Verification items for this drawing (mm, ordinates from the low corner). Round coordinates to 2 decimals unless told otherwise and drop trailing zeros. Order: outer loops, then holes, each group sorted by start corner. A loop starts at its lowest first (then second) coordinate and runs counter-clockwise, first axis right, second up. Notation, with made-up numbers: (61, 21) -> (106, 21) arc R17 cw to (106, 29) -> close; hole circle Ø2 at (35.5, 4). An arc over 180 degrees is marked (long way). Answer in a Markdown table with one row per item.
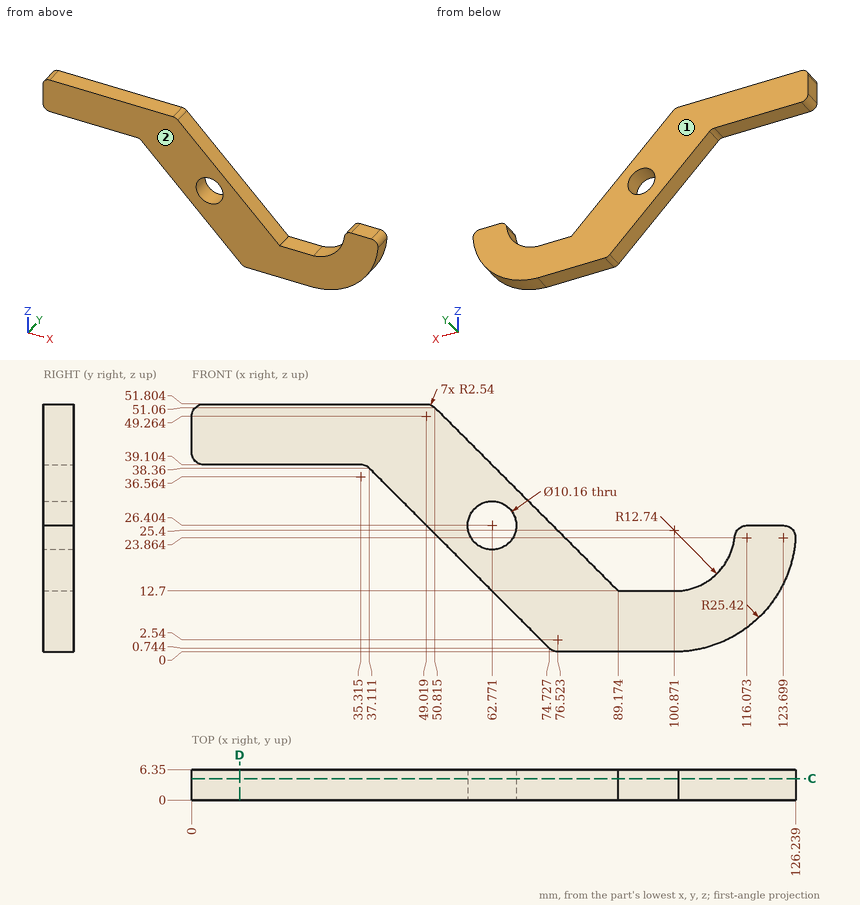
Item 1: Depth check by flat-ended pin: P1, Ø1, axis at y = 5, z = 41, coming from the -X side; P2, Ø1.5, axis at x = 15.5, y = 0.5, coming from the -Z side; P3, Ø11.5, axis at x = 62.77, z = 26.4, coming from the +Y side; P4, Ø1.5, axis at y = 1, z = 9.5, coming from the -X side. Enter the tip coordinate at first touch or a pass-through.
Result sheet:
| item | result |
|---|---|
| P1 | stops at x = 0 |
| P2 | stops at z = 39.1 |
| P3 | stops at y = 6.35 |
| P4 | stops at x = 65.22 |
Item 2: Mould release check, pull along Y, two halves, no side actions. Record for the marked faces 1 and 2: pulls with the +Y half, pulls with the -Y half, needs draft (parallel to the pull), parting line crosses it, or undercut.
Result sheet:
| item | result |
|---|---|
| face 1 | pulls with the +Y half |
| face 2 | pulls with the -Y half |
Item 3: Cross-section at D-D (x = 10). Record the boundary of the cut face in (y, z).
Result sheet:
| item | result |
|---|---|
| outline | (0, 39.1) -> (6.35, 39.1) -> (6.35, 51.8) -> (0, 51.8) -> close |
Item 4: Cross-section at C-C (y = 4.5). Record the boundary of the cut face in (x, z) (1 decimal).
Result sheet:
| item | result |
|---|---|
| outline | (0, 41.6) arc R2.5 ccw to (2.5, 39.1) -> (35.3, 39.1) arc R2.5 cw to (37.1, 38.4) -> (74.7, 0.7) arc R2.5 ccw to (76.5, 0) -> (101.9, 0) arc R25.4 ccw to (126.2, 23.7) arc R2.5 ccw to (123.7, 26.4) -> (116.1, 26.4) arc R2.5 ccw to (113.5, 24.1) arc R12.7 cw to (101.9, 12.7) -> (89.2, 12.7) -> (50.8, 51.1) arc R2.5 ccw to (49, 51.8) -> (2.5, 51.8) arc R2.5 ccw to (0, 49.3) -> close; hole circle Ø10.2 at (62.8, 26.4) |
Item 5: Scan lines: line 1 (Z direction, x = 61, y = 4) (1 decimal); line 2 (X direction, y = 5, z = 19) (1 decimal); line 3 (Z direction, x = 90, y = 4.25). Record each from-to range of solid material in increasing order. Write a range as [from, to].
Result sheet:
| item | result |
|---|---|
| line 1 | z = [14.5, 21.6], [31.2, 40.9] |
| line 2 | x = [56.5, 82.9], [111.9, 125.5] |
| line 3 | z = [0, 12.7] |
